Geometry: final body of the model. Coordinates: model frame, mm. A direction names the side the tool comes from. Coordinates: 2 decimals unless noted, no trailing zeros. Order: outer loops, then holes, each group sorted by start corner. A loop starts at its lowest first (then second) coordinate and runs counter-clockwise, first axis right, second up. Notation, with made-up numbers: M -24.75,57 L -17.75,57 A9 cw -17.75,74 Z; hole C -19.75,-14.75 d1. An arc over 180 degrees is marked long. Write item = value, one per line.
from build123d import *

# Parameters (mm, degrees)
BOSS_EXTRUDE1_DEPTH = 12.7
SKETCH2_R           = 2.675
CUT_EXTRUDE1_DEPTH  = 16.24
SKETCH3_W           = 7.62
SKETCH3_H           = 3.81
CUT_EXTRUDE2_DEPTH  = 96.8300001


with BuildPart() as part:
    # Sketch1 → Boss-Extrude1 (new body)
    with BuildSketch(Plane.XY):
        with BuildLine():
            Line((-47.915, 0), (47.915, 0))
            Line((47.915, 0), (47.915, -15.24))
            ThreePointArc((47.915, -15.24), (0, -10.434910675), (-47.915, -15.24))
            Line((-47.915, -15.24), (-47.915, 0))
        make_face()
    extrude(amount=BOSS_EXTRUDE1_DEPTH)

    # Sketch2 → Cut-Extrude1 (cut, through all)
    with BuildSketch(Plane(origin=(0, 0, 0), x_dir=(1, 0, 0), z_dir=(0, 1, 0))):
        with Locations((-40.915, -6.35)):
            Circle(SKETCH2_R)
        with Locations((40.915, -6.35)):
            Circle(SKETCH2_R)
    extrude(amount=-CUT_EXTRUDE1_DEPTH, mode=Mode.SUBTRACT)

    # Sketch3 → Cut-Extrude2 (cut, through all)
    with BuildSketch(Plane(origin=(47.915, 0, 0), x_dir=(0, 0, -1), z_dir=(1, 0, 0))):
        with Locations((-6.35, -13.335)):
            Rectangle(SKETCH3_W, SKETCH3_H)
    extrude(amount=-CUT_EXTRUDE2_DEPTH, mode=Mode.SUBTRACT)


solid = part.part
1) Section C-C, the plane x = 24. Return loops of the section in (y, z), and give its area (3 significant figures).
Numbers:
outline = M -11.63,0 L 0,0 L 0,12.7 L -11.63,12.7 L -11.63,10.16 L -11.43,10.16 L -11.43,2.54 L -11.63,2.54 Z
area = 146 mm²
2) Section B-B, the plane y = -8.5. Return loops of the section in (x, z) (3 decimals), and give its area (3 significant figures).
Numbers:
outline = M -47.915,0 L 47.915,0 L 47.915,12.7 L -47.915,12.7 Z; hole C -40.915,6.35 d5.35; hole C 40.915,6.35 d5.35
area = 1,170 mm²
3) Set-up query: faces 4 (the face through (-35, -11.43, 6)), 5 (the face through (38.243, -5.635, 6.232)). Return all of +Z, -Z, +X, -X, +Y, -Y with unobstructed straight access to the full face (end or side cutting, diameter ignored); none if empty.
Numbers:
face_4 = +X, -X, -Y
face_5 = +Y, -Y
4) Line query: L1, parallel to X at y = -8.75, z = 6.35 (3 decimals); L2, parallel to X at y = -10, z = 4.75 (3 decimals); L3, parallel to Y at x = 33.5, z = 8.5. Output: solid intervals per line, ascending.
Numbers:
L1 = -47.915 to -43.59, -38.24 to 38.24, 43.59 to 47.915
L2 = -47.915 to -43.059, -38.771 to 38.771, 43.059 to 47.915
L3 = -11.43 to 0
5) Section A-A, the plane z = 6.35. Return loops of the section in (x, y) (3 decimals).
Numbers:
outline = M -47.915,-11.43 L -43.59,-11.43 L -43.59,0 L -47.915,0 Z; M -38.24,-11.43 L -21.892,-11.43 A241.3 cw 21.892,-11.43 L 38.24,-11.43 L 38.24,0 L -38.24,0 Z; M 43.59,-11.43 L 47.915,-11.43 L 47.915,0 L 43.59,0 Z
6) Mould query, pull axis X, two halves, no side actions, for faces 1 (the face through (-47.915, -8, 6)), 2 (the face through (0.675, -10.436, 6.261)), 3 (the face through (-41, -13, 2.54)). Classes: pulls with the +X half, pulls with the -X half, needs draft (parallel to the pull), parting line crosses it, or undercut.
Numbers:
face_1 = pulls with the -X half
face_2 = undercut
face_3 = needs draft
7) Pin query (flat end, axial travel): pin 1 (3 mm diameter, centred on x = 11, y = -12.5, fed in from -Z) (3 decimals); pin 2 (2.5 mm diameter, centred on x = -35.5, z = 8, fed in from -Y); pin 3 (6 mm diameter, centred on x = 41, z = 7.5, fed in from -Y); pin 4 (1 mm diameter, centred on x = -13.5, z = 10, fed in from -Y). Return the tip coordinate at first contact, or that it passes through.
Numbers:
pin_1 = through
pin_2 = -11.43
pin_3 = -14.19
pin_4 = -10.84
8) Section D-D, the plane x = -25. Return loops of the section in (y, z).
Numbers:
outline = M -11.73,0 L 0,0 L 0,12.7 L -11.73,12.7 L -11.73,10.16 L -11.43,10.16 L -11.43,2.54 L -11.73,2.54 Z
